Input: part model. Units: mm. Frame: model coordinates. Face numbers are marked on the shaded views. A direction names the side the tool comes from. Round coordinates to 2 decimals unless told otherwise and drop trailing zeros. Loops run counter-clockwise (first coordinate to the right, second up) from the corner with the lowest first, then second, coordinate; pieces in that order, holes last. Notation, with made-up numbers: (78.25, -31.75) -> (120.25, -31.75) arc R7 cw to (120.25, -26.75) -> close; hole circle Ø10 at (62, 63). An arc over 180 degrees is marked (long way). Answer in a Markdown table with one row per item. Add a question column.
Q1. Ray query, L1, parallel to X at y = 24.5, z = -12.5; L2, parallel to Y at x = 37.5, z = 14; L3, parallel to Y at x = -24, z = -18. Return the intervals inside material, ascending. Write a range as from..to.
Q2. Section C-C, the plane x = -5. Output: boundary loops of the cut face in (y, z), and give its area (3 significant figures).
Q3. Mould query, pull axis Z, two halves, no side actions, for the marked faces 1, 2 and 3. Classes: pulls with the +Z half, pulls with the -Z half, needs draft (parallel to the pull), parting line crosses it, or undercut.
Q4. Section B-B, the plane y = -16.5. Output: boundary loops of the cut face in (x, z).
Q5. Section A-A, the plane z = 14. Output: boundary loops of the cut face in (x, y).
Q6. Pin query (flat end, axial travel): pin 1 (2 mm diameter, centred on x = 25.5, y = 4, fed in from -Z); pin 2 (20 mm diameter, centred on x = 23, y = 9, fed in from +Z); pin 3 (5 mm diameter, centred on y = -4.5, z = 14, fed in from -X). Return the tip coordinate at first contact, or that it passes through.
Q7. Section D-D, the plane z = 9. Output: boundary loops of the cut face in (x, y), and give its area (3 significant figures).
Q8. Reachability of the marked faces 4, 5 and 6 from +Z, -Z, +X, -X, +Y, -Y: full face, straight path, thin tool, end or side. Return the list, or none.
```python
from build123d import *

# Parameters (mm, degrees)
F0_W          = 70
F0_H          = 40
F1_DEPTH      = 40
F1_DEPTH_BACK = 40
F2_W          = 40
F2_H          = 30
F3_DEPTH      = 8
F5_DEPTH      = 40
F6_W          = 40
F6_H          = 20
F7_DEPTH      = 25
F9_DEPTH      = 25
F10_W         = 80
F10_H         = 40
F11_DEPTH     = 35
F13_DEPTH     = 25
F14_T4_DEPTH  = 76.2347538298
F14_T9_DEPTH  = 76.2347538298
F14_T14_DEPTH = 76.2347538298
F14_T19_DEPTH = 76.2347538298
F15_W         = 5
F15_H         = 30
F16_DEPTH     = 10


# Not quite as in the source:
# - a fillet or chamfer that OpenCascade refuses, or shapes differently, is made with other operations: its cross-section is extruded or revolved along the edge and cut away or added


with BuildPart() as f1:
    # F0 (on Right) → F1 (new body, two sides)
    with BuildSketch(Plane.YZ) as f1_sk:
        Rectangle(F0_W, F0_H)
    extrude(amount=F1_DEPTH)
    extrude(f1_sk.sketch, amount=-F1_DEPTH_BACK)

    # F2 (on face) → F3 (cut)
    with BuildSketch(Plane.XY.offset(20)):
        with Locations((20, -15)):
            Rectangle(F2_W, F2_H)
        with Locations((20, 15)):
            Rectangle(F2_W, F2_H)
    extrude(amount=-F3_DEPTH, mode=Mode.SUBTRACT)

    # F4 (on face) → F5 (cut)
    with BuildSketch(Plane.XY.offset(20)):
        Polygon((-40, 10), (-40, 0), (-20, 0), (-20, 15), (-35, 15), (-35, 10), align=None)
        Polygon((-20, 0), (-40, 0), (-40, -10), (-35, -10), (-35, -15), (-20, -15), align=None)
    extrude(amount=-F5_DEPTH, mode=Mode.SUBTRACT)

    # F6 (on face) → F7 (cut)
    with BuildSketch(Plane.XZ.offset(35)):
        with Locations((10, -10)):
            Rectangle(F6_W, F6_H)
    extrude(amount=-F7_DEPTH, mode=Mode.SUBTRACT)

    # F8 (on face) → F9 (join)
    with BuildSketch(Plane.XZ.offset(10)):
        with BuildLine():
            Line((0, -20), (20, -20))
            ThreePointArc((20, -20), (10, -10), (0, -20))
        make_face()
        with BuildLine():
            ThreePointArc((0, -20), (10, -30), (20, -20))
            Line((20, -20), (0, -20))
        make_face()
    extrude(amount=F9_DEPTH)

    # F10 (on face) → F11 (cut)
    with BuildSketch(Plane(origin=(0, 35, 0), x_dir=(-1, 0, 0), z_dir=(0, 1, 0))):
        Rectangle(F10_W, F10_H)
    extrude(amount=-F11_DEPTH, mode=Mode.SUBTRACT)

    # F12: F1 across plane


with BuildPart() as f1_1:
    add(f1.part)
    add(f1.part.mirror(Plane.XZ))

    # F13 (add): a face of the model
    f13_faces = [f1_1.faces().sort_by_distance(p)[0] for p in [
        (10, -10, -24.2441318158),
    ]]
    extrude(f13_faces, amount=F13_DEPTH)

    # F14: fillet of radius 20.5 on 4 edges, made by hand


with BuildPart() as f14_tool2:
    # F14_s3 → F14_t4 (new body)
    with BuildSketch(Plane.XZ.offset(-35)):
        with BuildLine():
            ThreePointArc((30, -20), (23.8239195314, -5.8285992489), (9.5060984681, 0))
            Line((9.5060984681, 0), (30, 0))
            Line((30, 0), (30, -20))
        make_face()
    extrude(amount=F14_T4_DEPTH)

    split(bisect_by=Plane.XZ.offset(35), keep=Keep.BOTTOM)


with BuildPart() as f1_2:
    add(f1_1.part)

    # F14_t1: union F14_tool2
    add(f14_tool2.part)


with BuildPart() as f14_tool7:
    # F14_s8 → F14_t9 (new body)
    with BuildSketch(Plane.XZ.offset(-35)):
        with BuildLine():
            ThreePointArc((10.4939015319, 0), (-3.8239195314, -5.8285992489), (-10, -20))
            Line((-10, -20), (-10, 0))
            Line((-10, 0), (10.4939015319, 0))
        make_face()
    extrude(amount=F14_T9_DEPTH)

    split(bisect_by=Plane.XZ.offset(35), keep=Keep.BOTTOM)


with BuildPart() as f1_3:
    add(f1_2.part)

    # F14_t6: union F14_tool7
    add(f14_tool7.part)


with BuildPart() as f14_tool12:
    # F14_s13 → F14_t14 (new body)
    with BuildSketch(Plane.XZ.offset(35)):
        with BuildLine():
            ThreePointArc((30, -20), (23.8239195314, -5.8285992489), (9.5060984681, 0))
            Line((9.5060984681, 0), (30, 0))
            Line((30, 0), (30, -20))
        make_face()
    extrude(amount=-F14_T14_DEPTH)

    split(bisect_by=Plane.XZ.offset(-35), keep=Keep.TOP)


with BuildPart() as f1_4:
    add(f1_3.part)

    # F14_t11: union F14_tool12
    add(f14_tool12.part)


with BuildPart() as f14_tool17:
    # F14_s18 → F14_t19 (new body)
    with BuildSketch(Plane.XZ.offset(35)):
        with BuildLine():
            ThreePointArc((-10, -20), (-3.8239195314, -5.8285992489), (10.4939015319, 0))
            Line((10.4939015319, 0), (-10, 0))
            Line((-10, 0), (-10, -20))
        make_face()
    extrude(amount=-F14_T19_DEPTH)

    split(bisect_by=Plane.XZ.offset(-35), keep=Keep.TOP)


with BuildPart() as f1_5:
    add(f1_4.part)

    # F14_t16: union F14_tool17
    add(f14_tool17.part)

    # F15 (on face) → F16 (cut)
    with BuildSketch(Plane.XY.offset(20)):
        with Locations((-17.5, 0)):
            Rectangle(F15_W, F15_H)
    extrude(amount=-F16_DEPTH, mode=Mode.SUBTRACT)


solid = f1_5.part
```
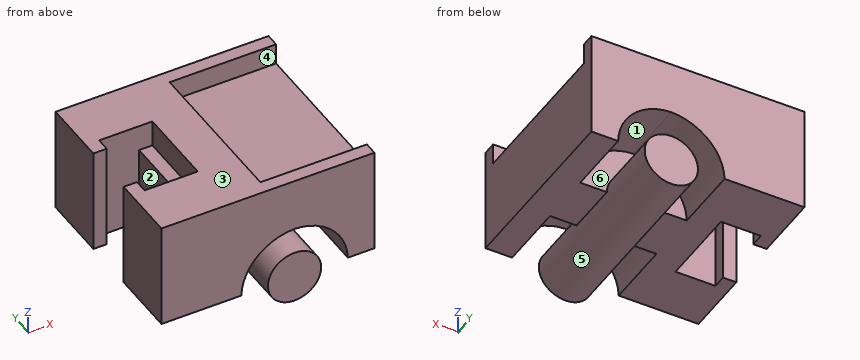
Answer block:
| question | item | result |
|---|---|---|
| 1 | L1 | -40..-8.38, 3.39..16.61, 28.38..40 |
| 1 | L2 | -35..-30, 30..35 |
| 1 | L3 | -35..-15, 15..35 |
| 2 | outline | (-35, -7.08) -> (-10, -7.08) -> (-10, -20) -> (10, -20) -> (10, -7.08) -> (35, -7.08) -> (35, 20) -> (-35, 20) -> close |
| 2 | area | 2,150 mm^2 |
| 3 | face 1 | undercut |
| 3 | face 2 | needs draft |
| 3 | face 3 | pulls with the +Z half |
| 4 | outline | (-40, -20) -> (-10, -20) arc R20.5 cw to (10, -0.01) arc R20.5 cw to (30, -20) -> (40, -20) -> (40, 12) -> (0, 12) -> (0, 20) -> (-40, 20) -> close; circle Ø20 at (10, -20) |
| 5 | outline | (-40, -35) -> (40, -35) -> (40, -30) -> (0, -30) -> (0, 30) -> (40, 30) -> (40, 35) -> (-40, 35) -> (-40, 10) -> (-35, 10) -> (-35, 15) -> (-15, 15) -> (-15, -15) -> (-35, -15) -> (-35, -10) -> (-40, -10) -> close |
| 6 | pin 1 | z = -20 |
| 6 | pin 2 | z = 12 |
| 6 | pin 3 | x = -15 |
| 7 | outline | (-40, -35) -> (40, -35) -> (40, 35) -> (-40, 35) -> (-40, 10) -> (-35, 10) -> (-35, 15) -> (-20, 15) -> (-20, -15) -> (-35, -15) -> (-35, -10) -> (-40, -10) -> close |
| 7 | area | 5,050 mm^2 |
| 8 | face 4 | +Z, +X |
| 8 | face 5 | none |
| 8 | face 6 | +Y |
